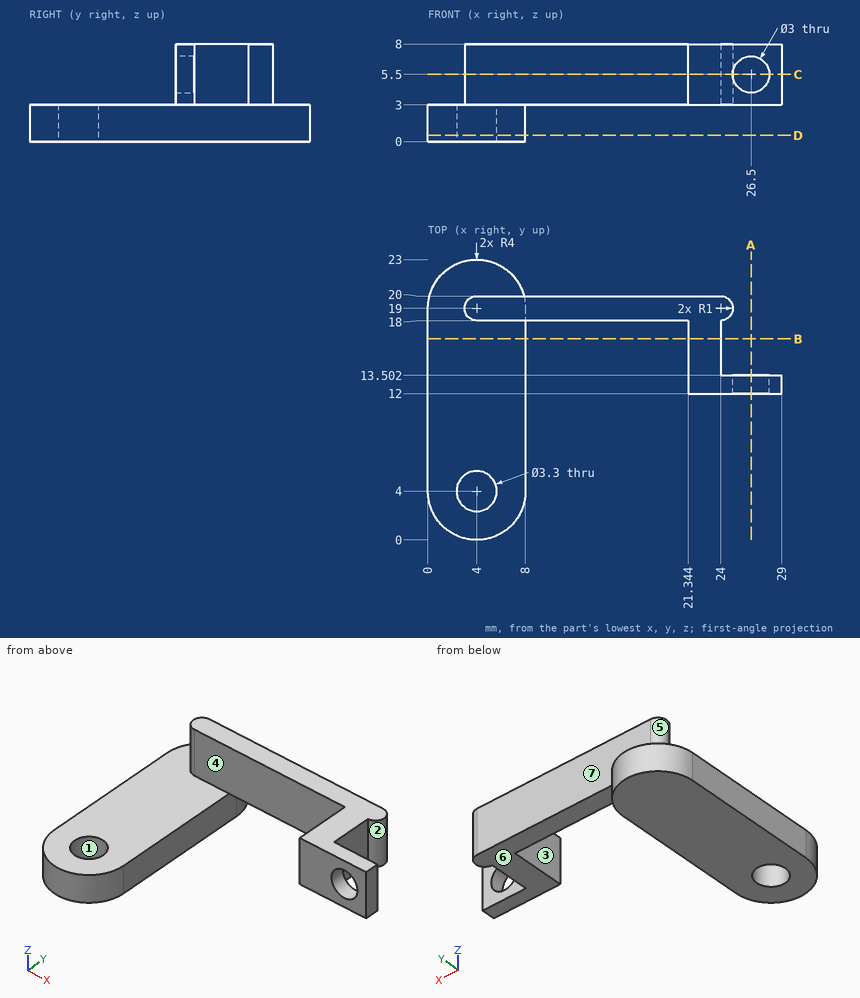
Geometry check sheet. Reference: drawing and pictorial views, mm from the part's lowest x, y, z. A direction names the side the tool comes from. Round coordinates to 2 decimals unless told otherwise and drop trailing zeros. Order: outer loops, then holes, each group sorted by start corner. A loop starts at its lowest first (then second) coordinate and runs counter-clockwise, first axis right, second up.
Q1. Cross-section at A-A, the plane x = 26.5. Enter the section's corners in (y, z).
Filled sheet:
outline: (12, 3) - (13.5, 3) - (13.5, 4) - (12, 4) - close; (12, 7) - (13.5, 7) - (13.5, 8) - (12, 8) - close
Q2. Depth check by flat-ended pin: P1, Ø2.5, axis at x = 9.5, z = 6, coming from the -Y side; P2, Ø2.5, axis at x = 26, z = 5, coming from the -Y side; P3, Ø1.5, axis at x = 16.5, z = 4, coming from the +Y side. Enter the tip coordinate at first touch or a pass-through.
Filled sheet:
P1: stops at y = 18
P2: stops at y = 12
P3: stops at y = 20
Q3. Cross-section at C-C, the plane z = 5.5. Enter the section's corners in (x, y).
Filled sheet:
outline: (4, 18) - (21.34, 18) - (21.34, 12) - (25, 12) - (25, 13.5) - (24, 13.5) - (24, 18) arc R1 ccw to (24, 20) - (4, 20) arc R1 ccw to start; (28, 12) - (29, 12) - (29, 13.5) - (28, 13.5) - close
Q4. Draft check along X on the marked faces 1, 2 and 3. Enter one of: pulls with the +X half, pulls with the -X half, needs draft (parallel to the pull), parting line crosses it, or undercut.
Filled sheet:
face 1: undercut
face 2: pulls with the +X half
face 3: pulls with the -X half
Q5. Cross-section at D-D, the plane z = 0.5. Enter the section's corners in (x, y), plus the area to 3 significant figures.
Filled sheet:
outline: (0, 4) arc R4 ccw to (8, 4) - (8, 19) arc R4 ccw to (0, 19) - close; hole circle Ø3.3 at (4, 4)
area: 162 mm2
Q6. Scan lines: L1, parallel to Y at x = 4, z = 1.05; L2, parallel to X at y = 13.1, z = 5.5; L3, parallel to Y at x = 4.5, z = 4. Record each from-to range of solid material in increasing order.
Filled sheet:
L1: y = 0 to 2.35, 5.65 to 23
L2: x = 21.34 to 25, 28 to 29
L3: y = 18 to 20
Q7. Cross-section at B-B, the plane y = 16.5. Enter the section's corners in (x, z), plus the area to 3 significant figures.
Filled sheet:
outline: (0, 0) - (8, 0) - (8, 3) - (0, 3) - close; (21.34, 3) - (24, 3) - (24, 8) - (21.34, 8) - close
area: 37.3 mm2
Q8. Set-up check for the marked faces 4, 5, 6 and 7: record each of +Z, -Z, +X, -X, +Y, -Y from which the full face is reachable in a straight line by a thin tool's end or side.
Filled sheet:
face 4: +Z, -X, -Y
face 5: +Z, -X
face 6: -Z, +X, +Y, -Y
face 7: +Z, +X, -X, +Y
